Design review of the part built by this model. Coordinates are the model's own, in mm. Face numbers are marked on the shaded views. A direction names the side the tool comes from. Give positions to 0.01 mm unless a question says otherwise; leave off trailing zeros. Loops run counter-clockwise (first coordinate to the right, second up) from the corner with the lowest first, then second, coordinate; pieces in that order, holes last. Notation, with made-up numbers: M -20.5,8.5 L 33.5,8.5 A16 ccw 33.5,39.5 Z; hole C -33,31.5 d11. An arc over 180 degrees is marked long. Use a Markdown table: item, result. Add a question column.
(1) Draft analysis for pull direction Z (two halves, no side actions). For the marked faces 3, 4, 5 and 6, state which applies: pulls with the +Z half, pulls with the -Z half, needs draft (parallel to the pull), parting line crosses it, or undercut.
(2) For probe 1 along X at (y, z) = (-0.65, -10.3); probe 2 along Z at (x, y) = (80.5, 3.5); probe 3 along Z at (x, y) = (60.45, -0.75), list the stretches that pass through material, from the lowest coordinate up.
(3) Add section D-D, the plane z = -1. Give the boundary of the cut face in (x, y), then the cut area to 3 significant figures.
(4) Add section B-B, the plane y = 3. Give the boundary of the cut face in (x, z), then the cut area to 3 significant figures.
(5) Insertion check: pin 1 Ø3 at (x, y) = (82.5, 7.5) entering from +Z; pin 2 Ø1.5 at (y, z) = (5, -1.5) entering from +X; pin 3 Ø1.8 at (y, z) = (2, 1) entering from +X; pin 4 Ø1.7 at (x, y) = (82.5, 7) entering from -Z. Each pin has a flat end and moves straight along its axis. Give the tip position at first contact, or say it passes through.
(6) Add section A-A, the plane x = 20.15. Give the boundary of the cut face in (y, z), then the cut area to 3 significant figures.
(7) Add section C-C, the plane x = 55. Give the boundary of the cut face in (y, z), then the cut area to 3 significant figures.
(8) For the marked faces 1 and 2, list the 3-axis set-ups (+Z, -Z, +X, -X, +Y, -Y) from which the entire face can be reached by the end or side of a thin tool; tool diameter is ignored.
```python
from build123d import *

# Parameters (mm, degrees)
SKETCH1_W           = 88.22
SKETCH1_H           = 28.2
SKETCH1_R           = 2.5
BOSS_EXTRUDE1_DEPTH = 1
SKETCH1_3_W         = 3.81
SKETCH1_3_H         = 5
BOSS_EXTRUDE2_DEPTH = 10.16
SKETCH1_4_W         = 80.6
SKETCH1_4_H         = 1.6
BOSS_EXTRUDE3_DEPTH = 6
BOSS_EXTRUDE4_DEPTH = 5
FILLET1_R           = 7
FILLET2_R           = 2
CHAMFER1_SIZE       = 0.6


with BuildPart() as part:
    # Sketch1 → Boss-Extrude1 (new body)
    with BuildSketch(Plane(origin=(0, 0, 0), x_dir=(1, 0, 0), z_dir=(0, 1, 0))):
        with Locations((40.3, 10.3)):
            Rectangle(SKETCH1_W, SKETCH1_H)
        with Locations((20.15, 10.3)):
            Circle(SKETCH1_R, mode=Mode.SUBTRACT)
        with Locations((60.45, 10.3)):
            Circle(SKETCH1_R, mode=Mode.SUBTRACT)
    extrude(amount=-BOSS_EXTRUDE1_DEPTH)

    # Sketch1<3> → Boss-Extrude2 (add)
    with BuildSketch(Plane(origin=(0, 0, 0), x_dir=(1, 0, 0), z_dir=(0, 1, 0))):
        with Locations((-1.905, 10.3)):
            Rectangle(SKETCH1_3_W, SKETCH1_3_H)
        with Locations((82.505, 10.3)):
            Rectangle(SKETCH1_3_W, SKETCH1_3_H)
    extrude(amount=BOSS_EXTRUDE2_DEPTH)

    # Sketch1<4> → Boss-Extrude3 (add)
    with BuildSketch(Plane(origin=(0, 0, 0), x_dir=(1, 0, 0), z_dir=(0, 1, 0))):
        with Locations((40.3, -0.8)):
            Rectangle(SKETCH1_4_W, SKETCH1_4_H)
        with Locations((40.3, 21.4)):
            Rectangle(SKETCH1_4_W, SKETCH1_4_H)
    extrude(amount=BOSS_EXTRUDE3_DEPTH)

    # Sketch2 → Boss-Extrude4 (add)
    with BuildSketch(Plane.XY.offset(-7.8)):
        Polygon((0, 10.16), (1.927427041, 8.905), (0, 7.16), align=None)
    boss_extrude4 = extrude(amount=-BOSS_EXTRUDE4_DEPTH)

    # Mirror1: Boss-Extrude4 across plane
    add(boss_extrude4.mirror(Plane.ZY.offset(-40.3)))

    # Fillet1
    fillet1_edges = [part.edges().sort_by_distance(p)[0] for p in [
        (84.41, -0.5, 3.8),
        (-3.81, -0.5, 3.8),
        (-3.81, -0.5, -24.4),
        (84.41, -0.5, -24.4),
    ]]
    fillet(fillet1_edges, radius=FILLET1_R)

    # Fillet2
    fillet2_edges = [part.edges().sort_by_distance(p)[0] for p in [
        (0, 0, -10.3),
        (-1.905, 0, -12.8),
        (-1.905, 0, -7.8),
        (82.505, 0, -7.8),
        (80.6, 0, -10.3),
        (82.505, 0, -12.8),
    ]]
    fillet(fillet2_edges, radius=FILLET2_R)

    # Chamfer1
    chamfer1_edges = [part.edges().sort_by_distance(p)[0] for p in [
        (17.65, 0, -10.3),
        (57.95, 0, -10.3),
    ]]
    chamfer(chamfer1_edges, length=CHAMFER1_SIZE)


solid = part.part
```
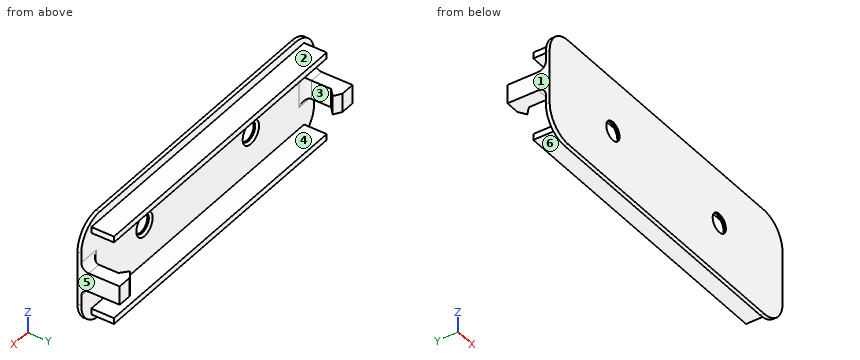
Established:
| question | item | result |
|---|---|---|
| 1 | face 3 | undercut |
| 1 | face 4 | undercut |
| 1 | face 5 | needs draft |
| 1 | face 6 | pulls with the -Z half |
| 2 | probe 1 | -3.81 to 17.65, 22.65 to 57.95, 62.95 to 84.41 |
| 2 | probe 2 | -22.2 to -20.6, 0 to 1.6 |
| 2 | probe 3 | -24.4 to -12.8, -7.8 to 3.8 |
| 3 | outline | M -3.46,-1 L 84.06,-1 L 84.06,0 L -3.46,0 Z |
| 3 | area | 87.5 mm^2 |
| 4 | outline | M -3.81,-12.8 L 0,-12.8 L 0,-7.8 L -3.81,-7.8 Z; M 0,-22.2 L 80.6,-22.2 L 80.6,-20.6 L 0,-20.6 Z; M 0,0 L 80.6,0 L 80.6,1.6 L 0,1.6 Z; M 80.6,-12.8 L 84.41,-12.8 L 84.41,-7.8 L 80.6,-7.8 Z |
| 4 | area | 296 mm^2 |
| 5 | pin 1 | z = -7.8 |
| 5 | pin 2 | through |
| 5 | pin 3 | x = 80.6 |
| 5 | pin 4 | z = -12.8 |
| 6 | outline | M -1,-24.4 L 0,-24.4 L 0,-22.2 L 6,-22.2 L 6,-20.6 L 0,-20.6 L 0,-13.4 L -0.6,-12.8 L -1,-12.8 Z; M -1,-7.8 L -0.6,-7.8 L 0,-7.2 L 0,0 L 6,0 L 6,1.6 L 0,1.6 L 0,3.8 L -1,3.8 Z |
| 6 | area | 42.0 mm^2 |
| 7 | outline | M -1,-24.4 L 0,-24.4 L 0,-22.2 L 6,-22.2 L 6,-20.6 L 0,-20.6 L 0,0 L 6,0 L 6,1.6 L 0,1.6 L 0,3.8 L -1,3.8 Z |
| 7 | area | 47.4 mm^2 |
| 8 | face 1 | +Z, -Z, -X, +Y, -Y |
| 8 | face 2 | +Z, +X, -X, +Y |
